Input: part model. Units: mm. Frame: model coordinates. A direction names the side the tool comes from. Give positions to 0.01 mm unless a question says otherwise; leave off trailing zeros. Loops run counter-clockwise (first coordinate to the right, second up) from the corner with the lowest first, then second, coordinate; pieces in that order, holes last. Notation, with made-up numbers: (77, 44.5) -> (83, 44.5) arc R29 cw to (83, 78.5) -> close; hole circle Ø6 at (-28, 78). An arc over 180 degrees is marked (long way). Answer in a Markdown table with one row per item. Add a question column.
Autodesk Inventor part; units mm, degrees
ref_plane "YZ Plane" through (0, 0, 0) normal (1, 0, 0) x (0, 1, 0)
ref_plane "XZ Plane" through (0, 0, 0) normal (0, 1, 0) x (-1, 0, 0)
ref_plane "XY Plane" through (0, 0, 0) normal (0, 0, 1) x (1, 0, 0)
sketch "Sketch1" plane through (0, 0, 0) normal (1, 0, 0) x (0, 1, 0)
  line L0 (0, 0) -> (25.4, 0)
  line L1 (25.4, 0) -> (25.4, -25.4)
  line L2 (25.4, -25.4) -> (0, -25.4)
  line L3 (0, -25.4) -> (0, 0)
  line L4 (3.175, -3.175) -> (22.225, -3.175)
  line L5 (22.225, -3.175) -> (22.225, -22.225)
  line L6 (22.225, -22.225) -> (3.175, -22.225)
  line L7 (3.175, -22.225) -> (3.175, -3.175)
  dimension "d0" = 25.4
  dimension "d1" = 25.4
  dimension "d2" = 19.05
  dimension "d3" = 19.05
  dimension "d4" = 3.175
  dimension "d5" = 3.175
extrude "Extrusion1" add sketch "Sketch1" along normal blind 152.4
sketch "Sketch2" plane through (0, 25.4, 0) normal (0, 1, 0) x (1, 0, 0)
  line L0 (0, 0) -> (0, 25.4)
  line L1 (0, 0) -> (152.4, 0)
  line L2 (152.4, 25.4) -> (152.4, 0)
  point P0 (38.1, 12.7)
  point P1 (114.3, 12.7)
  dimension "d8" = 38.1
  dimension "d9" = 12.7
  dimension "d10" = 12.7
  dimension "d11" = 38.1
hole "Hole1" at (38.1, 25.4, -12.7) at (114.3, 25.4, -12.7) direction (0, -1, 0) diameter 6.35 end through all
sketch "Sketch3" plane through (0, 0, 0) normal (0, 0, 1) x (1, 0, 0)
  line L0 (0, 0) -> (0, 25.4)
  line L1 (0, 0) -> (152.4, 0)
  line L2 (152.4, 25.4) -> (152.4, 0)
  point P0 (12.7, 17.4625)
  point P1 (136.525, 17.4625)
  dimension "d19" = 15.875
  dimension "d20" = 17.4625
  dimension "d21" = 12.7
  dimension "d22" = 17.4625
hole "Hole2" at (12.7, 17.4625, 0) at (136.525, 17.4625, 0) direction (0, 0, -1) diameter 4.3656 end through all
properties part number "1x1 pickup arm support" material "Aluminum 6061"
1) Material intervals for line 1 along X through (y, z) = (23.2, -12.7) (3 decimals); line 2 along Z through (x, y) = (130, 16.5) (3 decimals); line 3 along Y through (x, z) = (110.5, -6) (3 decimals), sorted ascending.
2) Section D-D on z = -6.5. Output: boundary loops of the cut face in (x, y) (3 decimals), and give its area (3 significant figures).
3) Section A-A on x = 38.1. Output: boundary loops of the cut face in (y, z) (3 decimals), and give its area (3 significant figures).
4) Reachability of faces 4 (the face through (138.656, 17.936, -1.61)), 5 (the face through (75, 13, -3.175)) from +Z, -Z, +X, -X, +Y, -Y: full face, straight path, thin tool, end or side. Return the list, or none.
5) Pull-direction query (X, two-part tool) for faces 1 (the face through (75, 22.225, -13)), 2 (the face through (0, 24, -13)), 3 (the face through (138.656, 17.936, -23.835)); classes: +X half, -X half, draft (parallel to the pull), parting line (faces both ways), or undercut.
6) Pin query (flat end, axial travel): pin 1 (8 mm diameter, centred on y = 11.5, z = -18.5, fed in from +X). Return the tip coordinate at first contact, or that it passes through.
7) Section B-B on y = 4.5. Output: boundary loops of the cut face in (x, z) (3 decimals), and give its area (3 significant figures).
8) Section C-C on z = -12.7. Output: boundary loops of the cut face in (x, y) (3 decimals).
Working result:
| question | item | result |
|---|---|---|
| 1 | line 1 | x = 0 to 34.925, 41.275 to 111.125, 117.475 to 152.4 |
| 1 | line 2 | z = -25.4 to -22.225, -3.175 to 0 |
| 1 | line 3 | y = 0 to 3.175, 22.225 to 25.4 |
| 2 | outline | (0, 0) -> (152.4, 0) -> (152.4, 3.175) -> (0, 3.175) -> close; (0, 22.225) -> (152.4, 22.225) -> (152.4, 25.4) -> (0, 25.4) -> close |
| 2 | area | 968 mm2 |
| 3 | outline | (0, -25.4) -> (25.4, -25.4) -> (25.4, -15.875) -> (22.225, -15.875) -> (22.225, -22.225) -> (3.175, -22.225) -> (3.175, -15.875) -> (0, -15.875) -> close; (0, -9.525) -> (3.175, -9.525) -> (3.175, -3.175) -> (22.225, -3.175) -> (22.225, -9.525) -> (25.4, -9.525) -> (25.4, 0) -> (0, 0) -> close |
| 3 | area | 242 mm2 |
| 4 | face 4 | +Z, -Z |
| 4 | face 5 | +X, -X |
| 5 | face 1 | draft |
| 5 | face 2 | -X half |
| 5 | face 3 | undercut |
| 6 | pin 1 | stops at x = 152.4 |
| 7 | outline | (0, -25.4) -> (152.4, -25.4) -> (152.4, -22.225) -> (0, -22.225) -> close; (0, -3.175) -> (152.4, -3.175) -> (152.4, 0) -> (0, 0) -> close |
| 7 | area | 968 mm2 |
| 8 | outline | (0, 0) -> (34.925, 0) -> (34.925, 3.175) -> (0, 3.175) -> close; (0, 22.225) -> (34.925, 22.225) -> (34.925, 25.4) -> (0, 25.4) -> close; (41.275, 0) -> (111.125, 0) -> (111.125, 3.175) -> (41.275, 3.175) -> close; (41.275, 22.225) -> (111.125, 22.225) -> (111.125, 25.4) -> (41.275, 25.4) -> close; (117.475, 0) -> (152.4, 0) -> (152.4, 3.175) -> (117.475, 3.175) -> close; (117.475, 22.225) -> (152.4, 22.225) -> (152.4, 25.4) -> (117.475, 25.4) -> close |
